```python
from build123d import *

# Parameters (mm, degrees)
BOSS_EXTRUDE1_DEPTH      = 20
BOSS_EXTRUDE1_DEPTH_BACK = 5
BOSS_EXTRUDE2_START      = -5
BOSS_EXTRUDE2_DEPTH      = 5
BOSS_EXTRUDE4_REACH      = 315.385


with BuildPart() as part:
    # Sketch1 → Boss-Extrude1 (new, two sides: drawn at the far end of the back side and taken through both)
    with BuildSketch(Plane.XY.offset(-BOSS_EXTRUDE1_DEPTH_BACK)):
        with BuildLine():
            Line((0, 25), (0, 17))
            ThreePointArc((0, 17), (-17, 0), (0, -17))
            Line((0, -17), (0, -25))
            ThreePointArc((0, -25), (-25, 0), (0, 25))
        make_face()
    extrude(amount=BOSS_EXTRUDE1_DEPTH + BOSS_EXTRUDE1_DEPTH_BACK)

    # Sketch2 → Boss-Extrude2 (add)
    with BuildSketch(Plane.XY.offset(BOSS_EXTRUDE2_START)):
        with BuildLine():
            Line((0, 25), (0, 77))
            Line((0, 77), (-65, 77))
            Line((-65, 77), (-65, 32.113081447))
            ThreePointArc((-65, 32.113081447), (-61.581037686, -38.262590053), (0, -72.5))
            Line((0, -72.5), (0, -25))
            ThreePointArc((0, -25), (-25, 0), (0, 25))
        make_face()
    extrude(amount=BOSS_EXTRUDE2_DEPTH)


with BuildPart() as body_2:
    # Mirror1: mirrored copy
    add(part.part.mirror(Plane.XY.offset(-140)))

    # Sketch3 → Boss-Extrude4 (add, up to next)
    with BuildSketch(Plane(origin=(0, 0, -5), x_dir=(-1, 0, 0), z_dir=(0, 0, -1)), mode=Mode.PRIVATE) as boss_extrude4_sk1:
        with BuildLine():
            Line((63, 31.642534665), (63, 77))
            Line((63, 77), (65, 77))
            Line((65, 77), (65, 32.113081447))
            ThreePointArc((65, 32.113081447), (61.581037686, -38.262590053), (0, -72.5))
            Line((0, -72.5), (0, -70.5))
            ThreePointArc((0, -70.5), (60.004369399, -37.009804823), (63, 31.642534665))
        make_face()
    boss_extrude4_tool1 = extrude(boss_extrude4_sk1.sketch, amount=BOSS_EXTRUDE4_REACH, mode=Mode.PRIVATE) - body_2.part

    add(part.part)  # Boss-Extrude4 merges part
    add(boss_extrude4_tool1.solids().sort_by_distance((-64.66152, 54.321267, -5))[0])


solid = body_2.part
```
Work out the finished part from the listing and answer in its coordinate system (mm). A direction names the side the tool comes from. Give positions to 0.01 mm unless a question says otherwise; leave off trailing zeros. Loops run counter-clockwise (first coordinate to the right, second up) from the corner with the lowest first, then second, coordinate; pieces in that order, holes last. Notation, with made-up numbers: (2.5, 64.25) -> (10.5, 64.25) arc R18 cw to (10.5, 72.25) -> close; hole circle Ø11 at (59.25, 71). An arc over 180 degrees is marked (long way). One line per question, with ' | ' between items. Start each with the question number.
1) Straight lines are drawn through the part: L1, parallel to Z at x = -38.5, y = 7.5; L2, parallel to Y at x = -7.5, z = 0.5; L3, parallel to X at y = 56.5, z = -7.5. For each, find the intervals that lie inside material, in ascending order.
2) Each of these flat-tipped pins is pushed along its axis until it touches: pin 1 (12 mm diameter, centred on y = 17, z = -89.5, fed in from +X); pin 2 (10 mm diameter, centred on x = -45, z = -259.5, fed in from -Y); pin 3 (1.5 mm diameter, centred on y = -36, z = -70.5, fed in from -X). Where does it stop, or does it pass through?
3) Determine the mould class of faces 4 (the face through (-24.994, -0.55, 9.86)), 5 (the face through (-59.47, -37.86, -138.11)), 6 (the face through (-18, 0, 20)) for opening direction Y: +Y half, -Y half, draft (parallel to the pull), parting line (faces both ways), or undercut.
4) Section C-C, the plane z = -266.5 is taken. Determine the outline of the cut face in (x, y).
5) Section D-D, the plane y = 0 is taken. Determine the outline of the cut face in (x, z), then the cut area to 4 significant figures.
6) Section A-A, the plane y = 52 is taken. Determine the outline of the cut face in (x, z).
7) For faces 1 (the face through (-63, 54, -138)), 2 (the face through (-37, 3, 0)), 3 (the face through (-37, 3, -280)), determine the directions among +Z, -Z, +X, -X, +Y, -Y from which every point of the face is accessible in a straight line to the end or side of a thin tool.
8) Section B-B, the plane x = -54.5 is taken. Determine the outline of the cut face in (y, z), then the cut area to 3 significant figures.
Resolved:
1) L1: -280 to -275, -5 to 0 | L2: -23.85 to -15.26, 15.26 to 23.85 | L3: -65 to -63
2) pin 1: x = -66.64 | pin 2: y = -60.47 | pin 3: x = -63.35
3) face 4: parting line | face 5: undercut | face 6: draft
4) outline: (-65, 32.11) arc R72.5 ccw to (0, -72.5) -> (0, -70.5) arc R70.5 cw to (-63, 31.64) -> (-63, 77) -> (-65, 77) -> close
5) outline: (-72.5, -280) -> (-25, -280) -> (-25, -300) -> (-17, -300) -> (-17, -275) -> (-70.5, -275) -> (-70.5, -5) -> (-17, -5) -> (-17, 20) -> (-25, 20) -> (-25, 0) -> (-72.5, 0) -> close | area: 1,415 mm2
6) outline: (-65, -280) -> (0, -280) -> (0, -275) -> (-63, -275) -> (-63, -5) -> (0, -5) -> (0, 0) -> (-65, 0) -> close
7) face 1: +X, +Y | face 2: +Z, -X | face 3: -Z, -X
8) outline: (-47.81, -280) -> (77, -280) -> (77, -275) -> (-44.72, -275) -> (-44.72, -5) -> (77, -5) -> (77, 0) -> (-47.81, 0) -> close | area: 2,080 mm2
